Here's how the part is built. I have some questions about the finished solid (model axes, mm). Face numbers are marked on the shaded views. Coordinates: 2 decimals unless noted, no trailing zeros. Order: outer loops, then holes, each group sorted by start corner. A loop starts at its lowest first (then second) coordinate and runs counter-clockwise, first axis right, second up. Notation, with made-up numbers: (81.25, 27) -> (91.25, 27) arc R13 ccw to (91.25, 31) -> close; hole circle Ø5 at (11.25, 25). An arc over 180 degrees is marked (long way). One line per item, written item: value. Start each with the question number.
Autodesk Inventor part; units mm, degrees
ref_plane "YZ Plane" through (0, 0, 0) normal (1, 0, 0) x (0, 1, 0)
ref_plane "XZ Plane" through (0, 0, 0) normal (0, 1, 0) x (-1, 0, 0)
ref_plane "XY Plane" through (0, 0, 0) normal (0, 0, 1) x (1, 0, 0)
sketch "Sketch1" plane through (0, 0, 0) normal (0, 1, 0) x (-1, 0, 0)
  circle A0 centre (0, 0) radius 7.62
  dimension "d0" = 15.24
extrude "Extrusion1" add sketch "Sketch1" along normal blind 25.4
sketch "Sketch2" plane through (0, 25.4, 0) normal (0, 1, 0) x (1, 0, 0)
  circle A0 centre (0, 0) radius 6.35
  dimension "d3" = 12.7
extrude "Extrusion2" cut sketch "Sketch2" against normal up to surface (25.4 mm away)
sketch "Sketch3" plane through (0, 25.4, 0) normal (0, 1, 0) x (1, 0, 0)
  circle A0 centre (0, 0) radius 6.3754
  dimension "d6" = 12.7508
extrude "Extrusion3" cut sketch "Sketch3" against normal blind 0.508
sketch "Sketch4" plane through (0, 0, 0) normal (0, -1, 0) x (1, 0, 0)
  circle A0 centre (0, 0) radius 6.3754
  dimension "d9" = 12.7508
extrude "Extrusion4" cut sketch "Sketch4" against normal blind 0.508
properties part number "brassbushing" material "Brass, Soft Yellow"
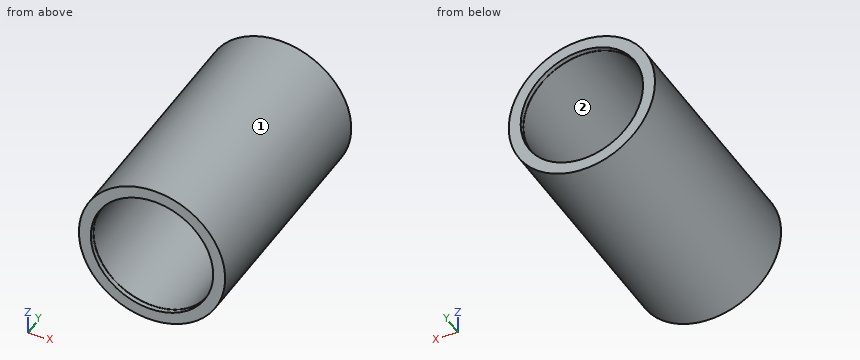
Q1. For P1, Ø4, axis at y = 14.5, z = 5, coming from the +X side; P2, Ø6, axis at y = 7.5, z = -4, coming from the +X side; P3, Ø4, axis at x = 2.5, y = 18.5, coming from the -Z side; P4, Ø6.5, axis at x = 0, z = 1, coming from the +Y side, each with a flat end and sliding along its axis, tell me the tip position at first contact or that it passes through.
Q2. I need wall thicknesses on line 1 (Z direction, x = 0, y = 0.25); line 2 (Z direction, x = -0.5, y = 15.75); line 3 (X direction, y = 15.75, z = -1.75). Which ranges of each line are inside material? Lowest first, please.
Q3. Imagine slicing it at C-C (y = 24). Write out the boundary of the cut face in (x, z).
Q4. If we mould it in two halves opening along X, with no side actions, what happens to the marked faces 1 and 2? For each: +X half, -X half, draft (parallel to the pull), parting line (faces both ways), or undercut.
Completed:
1. P1: stops at x = 7
1. P2: stops at x = 7.55
1. P3: stops at z = -7.6
1. P4: passes through
2. line 1: z = -7.62 to -6.38, 6.38 to 7.62
2. line 2: z = -7.6 to -6.33, 6.33 to 7.6
2. line 3: x = -7.42 to -6.1, 6.1 to 7.42
3. outline: circle Ø15.24 at (0, 0); hole circle Ø12.7 at (0, 0)
4. face 1: parting line
4. face 2: undercut
